```python
from build123d import *

# Parameters (mm, degrees)
F1_DEPTH = 6
F2_R     = 1.5
F3_DEPTH = 6.6
F4_R     = 3


with BuildPart() as f1:
    # F0 (on Front) → F1 (new body)
    with BuildSketch(Plane.XZ):
        Polygon((-5, -5), (5, -5), (5, 5), (5, 8.7), (-5, 8.7), (-5, 5), align=None)
        with BuildLine():
            ThreePointArc((1.852026, 2.1), (0, -2.8), (-1.852026, 2.1))
            Line((-1.852026, 2.1), (0, 2.1))
            Line((0, 2.1), (1.852026, 2.1))
        make_face(mode=Mode.SUBTRACT)
        Polygon((2.95, 4.1), (0, 4.1), (-2.95, 4.1), (-2.95, 6.7), (2.95, 6.7), align=None, mode=Mode.SUBTRACT)
    extrude(amount=F1_DEPTH)

    # F2 (on face) → F3 (cut, through all)
    with BuildSketch(Plane.XY.offset(8.7)):
        with Locations((0, -3)):
            Circle(F2_R)
    extrude(amount=-F3_DEPTH, mode=Mode.SUBTRACT)

    # F4
    f4_edges = [f1.edges().sort_by_distance(p)[0] for p in [
        (5, -3, -5),
        (-5, -3, -5),
    ]]
    fillet(f4_edges, radius=F4_R)


solid = f1.part
```
Read the model definition and answer for the solid it produces. Units are mm, in the model's axes. A direction names the side the tool comes from. Give positions to 0.01 mm unless a question says otherwise; leave off trailing zeros. Write each loop counter-clockwise with the first axis right and the second up, starting at its lowest first coordinate (ties: lowest second). Pieces come first, ordered by that corner, then holes. Notation, with made-up numbers: M 80,-31.75 L 103,-31.75 A34 ccw 103,1.25 Z; hole C 66,79.5 d3. An arc over 180 degrees is marked long. Put each result on its own line as item: value. Start each with the question number.
1. The part is cut by section B-B, the plane z = 0. Give the vertices of the cut face in (x, y).
2. The part is cut by section A-A, the plane x = 0. Give the vertices of the cut face in (y, z), and give its area (3 significant figures).
3. The part is cut by section D-D, the plane y = -3. Give the vertices of the cut face in (x, z), and give its area (3 significant figures).
4. The part is cut by section C-C, the plane y = -0.8. Give the vertices of the cut face in (x, z), and give its area (3 significant figures).
5. Consider line 1 along Y through (x, z) = (0, 7.5); line 2 along Z through (x, y) = (-1.25, -4.8); line 3 along Z through (x, y) = (-0.75, -1.2). Determine where each line is inside the solid, lowest interval first.
6. For a pull along Z with two mould halves and no side action, classify faces 4 (the flat face through (1.2, -1.6, 8.7)), 5 (the flat face through (5, -3, 3)), 6 (the cylindrical face through (0.1, -3, -2.8)) as released by +Z, released by -Z, zero draft, split by the parting line, or undercut.
7. Each of these flat-tipped pins is pushed along its axis until it touches: pin 1 Ø2.5 at (x, y) = (0, -3) entering from +Z; pin 2 Ø1.8 at (x, y) = (0, -3) entering from +Z; pin 3 Ø1 at (x, z) = (0, -0.5) entering from -Y. Where does it stop, or does it pass through?
8. Which of the six approach directions +Z, -Z, +X, -X, +Y, -Y give full straight-line access (tool end or side, diameter ignored) to faces 1 (the cylindrical face through (-0.195, -1.513, 7.714)), 2 (the flat face through (-2.95, -3, 5)), 3 (the flat face through (0, 0, 3))?
Final values:
1. outline: M -5,-6 L -2.8,-6 L -2.8,0 L -5,0 Z; M 2.8,-6 L 5,-6 L 5,0 L 2.8,0 Z
2. outline: M -6,-5 L 0,-5 L 0,-2.8 L -6,-2.8 Z; M -6,2.1 L -4.5,2.1 L -4.5,4.1 L -6,4.1 Z; M -6,6.7 L -4.5,6.7 L -4.5,8.7 L -6,8.7 Z; M -1.5,2.1 L 0,2.1 L 0,4.1 L -1.5,4.1 Z; M -1.5,6.7 L 0,6.7 L 0,8.7 L -1.5,8.7 Z
2. area: 25.2 mm²
3. outline: M -5,-2 A3 ccw -2,-5 L 2,-5 A3 ccw 5,-2 L 5,8.7 L 1.5,8.7 L 1.5,6.7 L 2.95,6.7 L 2.95,4.1 L 1.5,4.1 L 1.5,2.1 L 1.85,2.1 A2.8 cw long -1.85,2.1 L -1.5,2.1 L -1.5,4.1 L -2.95,4.1 L -2.95,6.7 L -1.5,6.7 L -1.5,8.7 L -5,8.7 Z
3. area: 82.9 mm²
4. outline: M -5,-2 A3 ccw -2,-5 L 2,-5 A3 ccw 5,-2 L 5,8.7 L -5,8.7 Z; hole M -2.95,4.1 L 2.95,4.1 L 2.95,6.7 L -2.95,6.7 Z; hole M -1.85,2.1 A2.8 ccw long 1.85,2.1 Z
4. area: 94.9 mm²
5. line 1: y = -6 to -4.5, -1.5 to 0
5. line 2: z = -5 to -2.51, 2.1 to 4.1, 6.7 to 8.7
5. line 3: z = -5 to -2.7, 2.1 to 4.1, 6.7 to 8.7
6. face 4: released by +Z
6. face 5: zero draft
6. face 6: undercut
7. pin 1: stops at z = -2.51
7. pin 2: stops at z = -2.65
7. pin 3: passes through
8. face 1: +Z
8. face 2: +Y, -Y
8. face 3: +Z, -Z, +X, -X, +Y
